CAD build for the part. Positions are in the model's coordinates, mm. Round coordinates to 2 decimals unless told otherwise and drop trailing zeros. Order: outer loops, then holes, each group sorted by start corner. A loop starts at its lowest first (then second) coordinate and runs counter-clockwise, first axis right, second up. Notation, with made-up numbers: M 11.5,41.25 L 48.5,41.25 A18 cw 48.5,71.25 Z; hole C -21,-3.75 d9. An arc over 180 degrees is marked long. Put each result on its own line as item: value.
```python
from build123d import *

# Parameters (mm, degrees)
SKETCH1_W                            = 47.5
SKETCH1_H                            = 18.5
BOSS_EXTRUDE1_DEPTH                  = 3
F_3_3_3_3_DIAMETER_HOLE1_D           = 3.3
F_3_3_3_3_DIAMETER_HOLE1_CSINK_D     = 3.35
F_3_3_3_3_DIAMETER_HOLE1_CSINK_ANGLE = 90


with BuildPart() as part:
    # Sketch1 → Boss-Extrude1 (new body)
    with BuildSketch(Plane(origin=(0, 0, 0), x_dir=(1, 0, 0), z_dir=(0, 1, 0))):
        Rectangle(SKETCH1_W, SKETCH1_H)
    extrude(amount=BOSS_EXTRUDE1_DEPTH)

    # Ø3.3 (3.3) Diameter Hole1 (through all)
    with Locations(Plane(origin=(0, 3, 0), x_dir=(1, 0, 0), z_dir=(0, 1, 0))):
        with Locations((0, 0), (21, -7), (-21, 7), (-21, -7), (21, 7)):
            CounterSinkHole(F_3_3_3_3_DIAMETER_HOLE1_D / 2, F_3_3_3_3_DIAMETER_HOLE1_CSINK_D / 2, counter_sink_angle=F_3_3_3_3_DIAMETER_HOLE1_CSINK_ANGLE)


solid = part.part
```
Item 1: Band-saw the part on A-A on x = 0. Give the cut face in (y, z) (3 decimals).
Answers below:
outline: M 0,-9.25 L 3,-9.25 L 3,-1.675 L 2.975,-1.65 L 0,-1.65 Z; M 0,1.65 L 2.975,1.65 L 3,1.675 L 3,9.25 L 0,9.25 Z
Item 2: Band-saw the part on D-D on y = 1.7. Give the cut face in (x, z).
Answers below:
outline: M -23.75,-9.25 L 23.75,-9.25 L 23.75,9.25 L -23.75,9.25 Z; hole C -21,-7 d3.3; hole C -21,7 d3.3; hole C 0,0 d3.3; hole C 21,-7 d3.3; hole C 21,7 d3.3
Item 3: Band-saw the part on C-C on z = 0. Give the cut face in (x, y) (3 decimals).
Answers below:
outline: M -23.75,0 L -1.65,0 L -1.65,2.975 L -1.675,3 L -23.75,3 Z; M 1.65,0 L 23.75,0 L 23.75,3 L 1.675,3 L 1.65,2.975 Z
Item 4: Probe line 1 along X through (y, z) = (1.85, 7); line 2 along Z through (x, y) = (-21, 1.2); line 3 along Z through (x, y) = (0, 1.2). List the from-to ranges inside material, lowest first. Write a range as [from, to].
Answers below:
line 1: [-23.75, -22.65], [-19.35, 19.35], [22.65, 23.75]
line 2: [-9.25, -8.65], [-5.35, 5.35], [8.65, 9.25]
line 3: [-9.25, -1.65], [1.65, 9.25]
Item 5: Band-saw the part on B-B on z = -7. Give the cut face in (x, y) (3 decimals), and give its area (3 significant figures).
Answers below:
outline: M -23.75,0 L -22.65,0 L -22.65,2.975 L -22.675,3 L -23.75,3 Z; M -19.35,0 L 19.35,0 L 19.35,2.975 L 19.325,3 L -19.325,3 L -19.35,2.975 Z; M 22.65,0 L 23.75,0 L 23.75,3 L 22.675,3 L 22.65,2.975 Z
area: 123 mm²
Item 6: Mould opens along Z. For faces 1 (the flat face through (0, 3, -2)), 2 (the flat face through (0, 1, -9.25)), 3 (the cylindrical face through (22.31, 1.47, 8)) say: pulls with the +Z half, pulls with the -Z half, needs draft (parallel to the pull), parting line crosses it, or undercut.
Answers below:
face 1: needs draft
face 2: pulls with the -Z half
face 3: undercut
